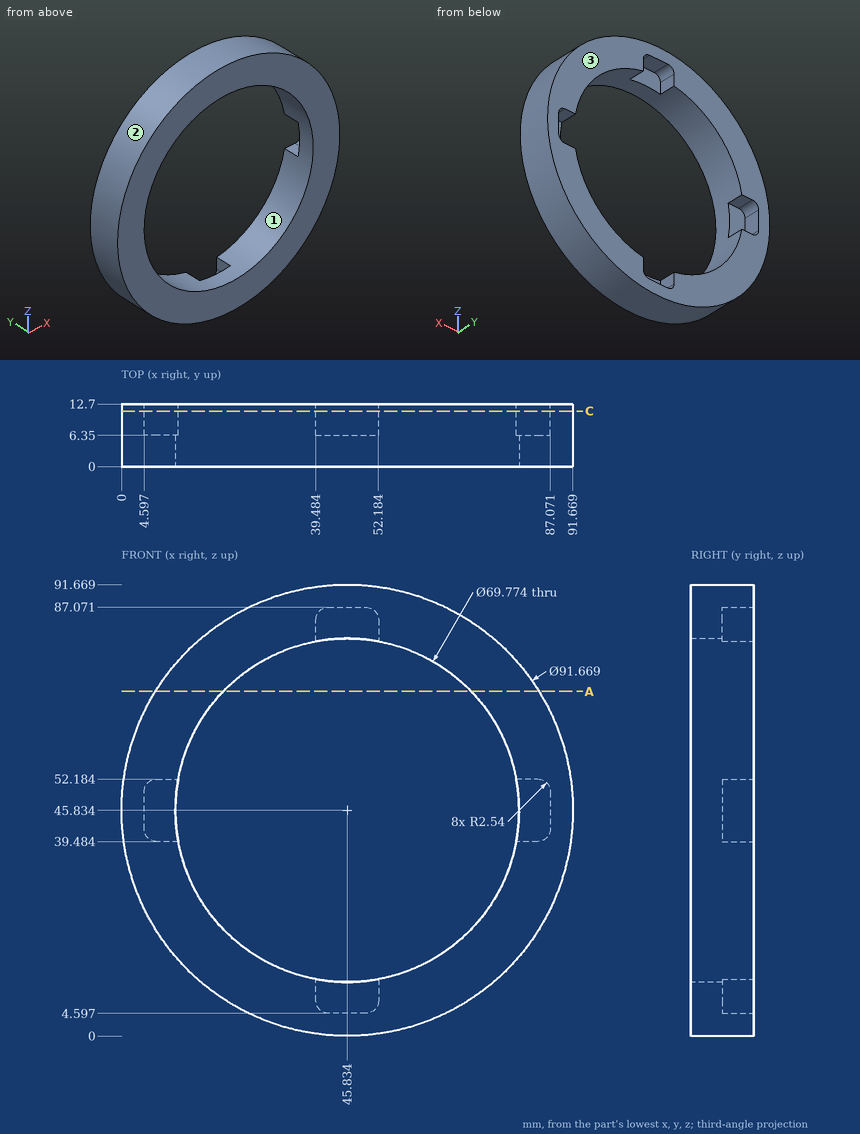
Answer from the drawing. Dimensions are ordinates in mm from the lowest x, y and z of the part. Coordinates: 2 decimals unless noted, no trailing zeros. Loops run counter-clockwise (first coordinate to the right, second up) from the corner with the lowest first, then second, coordinate; pieces in that order, holes last. Notation, with made-up numbers: (82.25, -40) -> (124.25, -40) arc R26 cw to (124.25, -6) -> close; hole circle Ø4 at (77, -36). An arc over 180 degrees is marked (long way). Answer as CSV lines item,"result".
Q1. The part is cut by section A-A on z = 70. Write down the section's boundary in (x, y), and give its area (3 significant figures).
Findings:
outline,"(6.89, 0) -> (20.67, 0) -> (20.67, 12.7) -> (6.89, 12.7) -> close; (71, 0) -> (84.78, 0) -> (84.78, 12.7) -> (71, 12.7) -> close"
area,"350 mm²"
Q2. The part is cut by section C-C on y = 11.25. Write down the section's boundary in (x, z) (1 decimal).
Findings:
outline,"circle Ø91.7 at (45.8, 45.8); hole (4.6, 42) arc R2.5 ccw to (7.1, 39.5) -> (11.5, 39.5) arc R34.9 ccw to (39.5, 11.5) -> (39.5, 7.1) arc R2.5 ccw to (42, 4.6) -> (49.6, 4.6) arc R2.5 ccw to (52.2, 7.1) -> (52.2, 11.5) arc R34.9 ccw to (80.1, 39.5) -> (84.5, 39.5) arc R2.5 ccw to (87.1, 42) -> (87.1, 49.6) arc R2.5 ccw to (84.5, 52.2) -> (80.1, 52.2) arc R34.9 ccw to (52.2, 80.1) -> (52.2, 84.5) arc R2.5 ccw to (49.6, 87.1) -> (42, 87.1) arc R2.5 ccw to (39.5, 84.5) -> (39.5, 80.1) arc R34.9 ccw to (11.5, 52.2) -> (7.1, 52.2) arc R2.5 ccw to (4.6, 49.6) -> close"
Q3. Find the intervals of material crossed by probe 1 along Z at (x, y) = (45.5, 4); probe 2 along Z at (x, y) = (43, 1.5) (1 decimal); probe 3 along X at (y, z) = (9.25, 81) (1 decimal), in increasing order.
Findings:
probe 1,"z = 0 to 10.95, 80.72 to 91.67"
probe 2,"z = 0.1 to 11.1, 80.6 to 91.6"
probe 3,"x = 16.4 to 39.5, 52.2 to 75.2"
Q4. Each of these flat-tipped pins is pushed along its axis until it touches: pin 1 (1.9 mm diameter, centred on y = 8.5, z = 45.5, fed in from +X); pin 2 (3.5 mm diameter, centred on x = 83, y = 11, fed in from +Z); pin 3 (5.5 mm diameter, centred on x = 48.5, z = 8.5, fed in from +Y). Where does it stop, or does it pass through?
Findings:
pin 1,"stops at x = 91.67"
pin 2,"stops at z = 74.93"
pin 3,"stops at y = 6.35"
Q5. For a pull along X with two mould halves and no side action, classify the marked faces 1, 2 and 3 as +X half, -X half, draft (parallel to the pull), parting line (faces both ways), or undercut.
Findings:
face 1,"undercut"
face 2,"parting line"
face 3,"draft"
